Input: dimensioned drawing with shaded views. Units: mm. Origin: part minimum x, y, z. A direction names the side the tool comes from. Round coordinates to 2 decimals unless told otherwise and drop trailing zeros. Loops run counter-clockwise (first coordinate to the right, second up) from the corner with the lowest first, then second, coordinate; pieces in that order, holes last.
1) Section C-C, the plane z = 10.75. Return loops of the section in (x, y), and give its area (3 significant figures).
2) First-contact query: pin 1 (4 mm diameter, centred on x = 14.5, z = 4.5, fed in from -Y). Flat tip, straight axial feed; report the tip coordinate or a pass-through.
3) Section D-D, the plane y = 14.5. Return loops of the section in (x, z), and give its area (3 significant figures).
4) Section B-B, the plane x = 10. Return loops of the section in (y, z), and give its area (3 significant figures).
5) Access query for the marked faces 5 and 6. Directions: +Z, -Z, +X, -X, +Y, -Y. A direction counts if a zero-diameter tool reaches every point of the face in a straight line with its end or side. Return the directions, or none.
6) Draft query along Z for the marked faces 1, 2, 3 and 4. Return one class per face: pulls with the +Z half, pulls with the -Z half, needs draft (parallel to the pull), parting line crosses it, or undercut.
7) Ray query, line 1 along Z through (x, y) = (1, 27); line 2 along X through (y, z) = (10, 1); line 3 along Y through (x, z) = (6.5, 9.25). Return the intervals inside material, ascending.
8) Section A-A, the plane y = 28. Return loops of the section in (x, z).
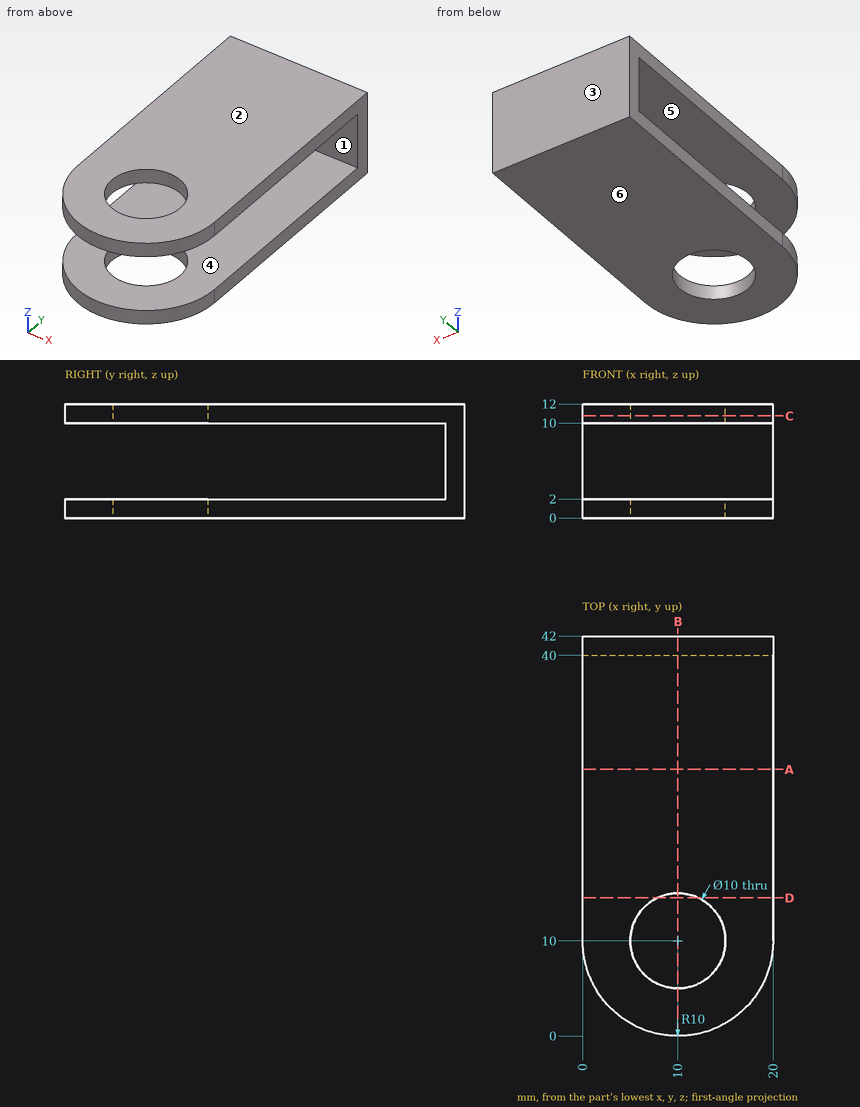
Final values:
1. outline: (0, 10) arc R10 ccw to (20, 10) - (20, 42) - (0, 42) - close; hole circle Ø10 at (10, 10)
1. area: 719 mm2
2. pin 1: stops at y = 40
3. outline: (0, 0) - (7.82, 0) - (7.82, 2) - (0, 2) - close; (0, 10) - (7.82, 10) - (7.82, 12) - (0, 12) - close; (12.18, 0) - (20, 0) - (20, 2) - (12.18, 2) - close; (12.18, 10) - (20, 10) - (20, 12) - (12.18, 12) - close
3. area: 62.6 mm2
4. outline: (0, 0) - (5, 0) - (5, 2) - (0, 2) - close; (0, 10) - (5, 10) - (5, 12) - (0, 12) - close; (15, 0) - (42, 0) - (42, 12) - (15, 12) - (15, 10) - (40, 10) - (40, 2) - (15, 2) - close
4. area: 144 mm2
5. face 5: +X, -X, -Y
5. face 6: -Z, +X, -X, +Y, -Y
6. face 1: undercut
6. face 2: pulls with the +Z half
6. face 3: needs draft
6. face 4: undercut
7. line 1: z = 0 to 2, 10 to 12
7. line 2: x = 0 to 5, 15 to 20
7. line 3: y = 40 to 42
8. outline: (0, 0) - (20, 0) - (20, 2) - (0, 2) - close; (0, 10) - (20, 10) - (20, 12) - (0, 12) - close
